Could you check a few things on this model? Use its own coordinates, in mm. A direction names the side the tool comes from. Give positions to 0.01 mm unless a question says otherwise; leave off trailing zeros. Order: outer loops, then holes, each group sorted by start corner. A loop starts at its lowest first (then second) coordinate and runs counter-clockwise, first axis right, second up. Notation, with made-up numbers: M 25.5,77 L 49.5,77 A7 ccw 49.5,81 Z; hole C -34,31 d3. An arc over 180 degrees is marked long. Return JSON: item names as keys, results as strings. Group by question number.
```python
from build123d import *

# Parameters (mm, degrees)
SKETCH_1_W          = 120
SKETCH_1_H          = 32
EXTRUDE_1_DEPTH     = 3
CUT_EXTRUDE_1_DEPTH = 69.066144301
SKETCH_2_3_W        = 27.5
SKETCH_2_3_H        = 3
EXTRUDE_2_DEPTH     = 3
SKETCH_3_W          = 3.2
SKETCH_3_H          = 32
EXTRUDE_3_DEPTH     = 72.5
EXTRUDE_4_DEPTH     = 3
SKETCH_5_W          = 3
SKETCH_5_H          = 3
CUT_EXTRUDE_2_DEPTH = 90.831181838
SKETCH_6_W          = 24.435270894
SKETCH_6_H          = 1
SKETCH_6_W_2        = 1
SKETCH_6_H_2        = 29
CUT_EXTRUDE_3_DEPTH = 1.5
SKETCH_7_W          = 1
SKETCH_7_H          = 71
CUT_EXTRUDE_4_DEPTH = 1.5
CUT_EXTRUDE_6_REACH = 91.831
SKETCH_7_5_W        = 1
SKETCH_7_5_H        = 22.499258378
CUT_EXTRUDE_7_DEPTH = 40.31507816
CUT_EXTRUDE_8_DEPTH = 1.5
SKETCH_10_R         = 0.35
CUT_EXTRUDE_9_DEPTH = 3


with BuildPart() as part:
    # 草图1 → 凸台-拉伸1 (new body)
    with BuildSketch(Plane(origin=(0, 0, 0), x_dir=(1, 0, 0), z_dir=(0, 1, 0))):
        Rectangle(SKETCH_1_W, SKETCH_1_H)
    extrude(amount=EXTRUDE_1_DEPTH)

    # 草图2 → 切除-拉伸1 (cut, through all)
    with BuildSketch(Plane(origin=(0, 0, -16), x_dir=(-1, 0, 0), z_dir=(0, 0, -1))):
        Polygon((-60, 0), (27, 0), (26.1, 3), (-60, 3), align=None)
    extrude(amount=-CUT_EXTRUDE_1_DEPTH, mode=Mode.SUBTRACT)

    # 草图2<3> → 凸台-拉伸2 (add)
    with BuildSketch(Plane(origin=(0, 0, -16), x_dir=(-1, 0, 0), z_dir=(0, 0, -1))):
        with Locations((43.05, 1.5)):
            Rectangle(SKETCH_2_3_W, SKETCH_2_3_H)
    extrude(amount=EXTRUDE_2_DEPTH)

    # 草图3 → 凸台-拉伸3 (add)
    with BuildSketch(Plane(origin=(0, 3, 0), x_dir=(1, 0, 0), z_dir=(0, 1, 0))):
        with Locations((-58.4, 0)):
            Rectangle(SKETCH_3_W, SKETCH_3_H)
    extrude(amount=EXTRUDE_3_DEPTH)

    # 草图4 → 凸台-拉伸4 (add)
    with BuildSketch(Plane.XY.offset(16)):
        Polygon((-11.98492184, 50.000741622), (-11.98492184, 72.5), (-17.98492184, 72.5), (-17.98492184, 50.882243247), (-32.364729106, 3), (-26.1, 3), align=None)
    extrude(amount=-EXTRUDE_4_DEPTH)

    # 草图5 → 切除-拉伸2 (cut, through all)
    with BuildSketch(Plane(origin=(-56.8, 0, 0), x_dir=(0, 0, -1), z_dir=(1, 0, 0))):
        with Locations((-14.5, 74)):
            Rectangle(SKETCH_5_W, SKETCH_5_H)
    extrude(amount=-CUT_EXTRUDE_2_DEPTH, mode=Mode.SUBTRACT)

    # 草图6 → 切除-拉伸3 (cut)
    with BuildSketch(Plane(origin=(0, 3, 0), x_dir=(1, 0, 0), z_dir=(0, 1, 0))):
        with Locations((-44.582364553, -14.5)):
            Rectangle(SKETCH_6_W, SKETCH_6_H)
        with Locations((-27.6, 1.5)):
            Rectangle(SKETCH_6_W_2, SKETCH_6_H_2)
    extrude(amount=-CUT_EXTRUDE_3_DEPTH, mode=Mode.SUBTRACT)

    # 草图7 → 切除-拉伸4 (cut)
    with BuildSketch(Plane(origin=(-56.8, 0, 0), x_dir=(0, 0, -1), z_dir=(1, 0, 0))):
        with Locations((-14.5, 37)):
            Rectangle(SKETCH_7_W, SKETCH_7_H)
    extrude(amount=-CUT_EXTRUDE_4_DEPTH, mode=Mode.SUBTRACT)

    # 切除-拉伸6: up to this plane
    cut_extrude_6_end = Plane(origin=(-29.077043909, 8.732303646, 13), z_dir=(0.9577429283961915, -0.2876255953615531, 0))
    # 草图7<4> → 切除-拉伸6 (cut, up to the surface)
    with BuildSketch(Plane(origin=(-56.8, 0, 0), x_dir=(0, 0, -1), z_dir=(1, 0, 0)), mode=Mode.PRIVATE) as cut_extrude_6_sk1:
        Polygon((-15, 3), (-15, 1.5), (-14, 1.5), (-14, 3), (-14, 50.000741622), (-15, 50.000741622), align=None)
    cut_extrude_6_tool1 = split(extrude(cut_extrude_6_sk1.sketch, amount=CUT_EXTRUDE_6_REACH, mode=Mode.PRIVATE), bisect_by=cut_extrude_6_end, keep=Keep.BOTH, mode=Mode.PRIVATE)
    add(cut_extrude_6_tool1.solids().sort_by_distance((-56.8, 25.750371, 14.5))[0], mode=Mode.SUBTRACT)

    # 草图7<5> → 切除-拉伸7 (cut)
    with BuildSketch(Plane(origin=(-56.8, 0, 0), x_dir=(0, 0, -1), z_dir=(1, 0, 0))):
        with Locations((-14.5, 61.250370811)):
            Rectangle(SKETCH_7_5_W, SKETCH_7_5_H)
    extrude(amount=CUT_EXTRUDE_7_DEPTH, mode=Mode.SUBTRACT)

    # 草图9 → 切除-拉伸8 (cut)
    with BuildSketch(Plane(origin=(0, 0, 13), x_dir=(-1, 0, 0), z_dir=(0, 0, -1))):
        Polygon((28.1, 1.5), (27.1, 1.5), (27.1, 3), (12.98492184, 50.000741622), (12.98492184, 72.5), (13.98492184, 72.5), (13.98492184, 50.000741622), (28.1, 3), align=None)
    extrude(amount=-CUT_EXTRUDE_8_DEPTH, mode=Mode.SUBTRACT)

    # 草图10 → 切除-拉伸9 (cut)
    with BuildSketch(Plane(origin=(0, 72.5, 0), x_dir=(1, 0, 0), z_dir=(0, 1, 0))):
        with Locations(Location((-14.98492184, -14.5, 0), (0, 0, 270))):
            Circle(SKETCH_10_R)
    extrude(amount=-CUT_EXTRUDE_9_DEPTH, mode=Mode.SUBTRACT)


solid = part.part
```
1. I need wall thicknesses on L1, parallel to X at y = 61, z = 13.5; L2, parallel to Z at x = -27.5, y = 17.5; L3, parallel to X at y = 50.5, z = 4. Which ranges of each line are inside material? Lowest first, please. Write a range as from..to.
2. Which directions (+Z, -Z, +X, -X, +Y, -Y) give clear straight access to the entire face, cutting with the end or side of a thin tool? Please do faces 1 (the flat face through (-24.07, 25.41, 14.51)), 2 (the flat face through (-59, 72.5, 15)), 3 (the flat face through (-28, 1, -16)), 4 (the flat face through (-25.074, 27.276, 13.507)).
3. Imagine slicing it at C-C, the plane z = -7. Please give me the cut outline in (x, y), plus the area to 3 significant figures.
4. For pin 1 (1.5 mm diameter, centred on x = -57.5, y = 73.5, fed in from +Z); pin 2 (1.1 mm diameter, centred on y = 46.5, z = 14.5, fed in from +X); pin 3 (2.5 mm diameter, centred on x = -15.5, z = 14, fed in from +Y), each with a flat end and sliding along its axis, tell me the tip position at first contact or that it passes through.
5. Imagine slicing it at B-B, the plane x = -36. Please give me the cut outline in (y, z), plus the area to 4 significant figures.
6. Imagine slicing it at D-D, the plane y = 13.5. Please give me the cut outline in (x, z).
7. Imagine slicing it at A-A, the plane y = 60. Please give me the cut outline in (x, z).
8. If we mould it in two halves opening along Z, with no side actions, what happens to faces 5 (the flat face through (-13.985, 61, 14)), 6 (the flat face through (-25, 26, 15)), 7 (the flat face through (-20, 38, 13))? For each: pulls with the +Z half, pulls with the -Z half, needs draft (parallel to the pull), parting line crosses it, or undercut.
Values:
{
 "1": {"L1": "x = -60..-56.8, -17.98..-13.98, -12.98..-11.98", "L2": "z = 13..14, 15..16", "L3": "x = -60..-56.8"},
 "2": {"face 1": "+Y", "face 2": "+Z, +X, -X, +Y", "face 3": "-Z, +X, +Y, -Y", "face 4": "+Z, -Z, +Y"},
 "3": {"outline": "M -60,0 L -27,0 L -26.1,3 L -27.1,3 L -27.1,1.5 L -28.1,1.5 L -28.1,3 L -56.8,3 L -56.8,75.5 L -60,75.5 Z", "area": "331 mm²"},
 "4": {"pin 1": "stops at z = 13", "pin 2": "stops at x = -12.87", "pin 3": "stops at y = 72.5"},
 "5": {"outline": "M 0,-19 L 3,-19 L 3,14 L 1.5,14 L 1.5,15 L 3,15 L 3,16 L 0,16 Z", "area": "103.5 mm²"},
 "6": {"outline": "M -60,-16 L -56.8,-16 L -56.8,14 L -58.3,14 L -58.3,15 L -56.8,15 L -56.8,16 L -60,16 Z; M -29.21,13 L -24.95,13 L -24.95,14.5 L -23.95,14.5 L -23.95,13 L -22.95,13 L -22.95,16 L -29.21,16 L -29.21,15 L -27.65,15 L -27.65,14 L -29.21,14 Z"},
 "7": {"outline": "M -60,-16 L -56.8,-16 L -56.8,14 L -58.3,14 L -58.3,15 L -56.8,15 L -56.8,16 L -60,16 Z; M -17.98,13 L -13.98,13 L -13.98,14.5 L -12.98,14.5 L -12.98,13 L -11.98,13 L -11.98,16 L -17.98,16 L -17.98,15 L -16.48,15 L -16.48,14 L -17.98,14 Z"},
 "8": {"face 5": "needs draft", "face 6": "undercut", "face 7": "pulls with the -Z half"}
}
